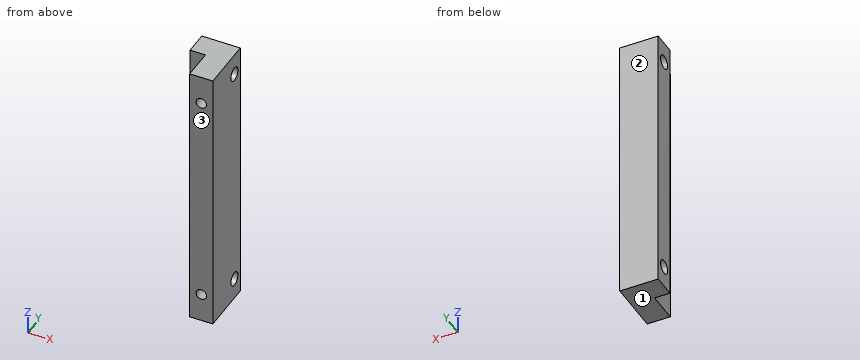
from build123d import *

# Parameters (mm, degrees)
AUFSATZ_LINEAR_AUSTRAGEN1_DEPTH = 89
M8_GEWINDEBOHRUNG1_D            = 6.8
M8_GEWINDEBOHRUNG1_DEPTH        = 18.25
M8_GEWINDEBOHRUNG1_TIP          = 2.042926105
F_9_0_9_DURCHMESSER_BOHRUNG1_D  = 9


with BuildPart() as part:
    # Skizze1 → Aufsatz-Linear austragen1 (new, symmetric)
    with BuildSketch(Plane.XY):
        Polygon((0, 0), (15, 0), (15, 35), (-10, 35), (-10, 20), (0, 20), align=None)
    extrude(amount=AUFSATZ_LINEAR_AUSTRAGEN1_DEPTH, both=True)

    # M8 Gewindebohrung1
    with Locations(Plane(origin=(0, 0, 0), x_dir=(-1, 0, 0), z_dir=(0, -1, 0))):
        with Locations((-7.5, -70), (-7.5, 70)):
            Hole(M8_GEWINDEBOHRUNG1_D / 2, depth=M8_GEWINDEBOHRUNG1_DEPTH)
            with Locations((0, 0, -(M8_GEWINDEBOHRUNG1_DEPTH + M8_GEWINDEBOHRUNG1_TIP / 2))):  # 118° drill point
                Cone(0, M8_GEWINDEBOHRUNG1_D / 2, M8_GEWINDEBOHRUNG1_TIP, mode=Mode.SUBTRACT)

    # Ø9.0 (9) Durchmesser Bohrung1 (through all)
    with Locations(Plane(origin=(15, 0, 0), x_dir=(0, 0, -1), z_dir=(1, 0, 0))):
        with Locations((-75, 27.5), (75, 27.5)):
            Hole(F_9_0_9_DURCHMESSER_BOHRUNG1_D / 2)


solid = part.part
Here's how the part is built. I have some questions about the finished solid (model axes, mm). Face numbers are marked on the shaded views. Round coordinates to 2 decimals unless told otherwise and drop trailing zeros. Order: outer loops, then holes, each group sorted by start corner. A loop starts at its lowest first (then second) coordinate and runs counter-clockwise, first axis right, second up. Notation, with made-up numbers: M -30,59.5 L 15,59.5 A19 cw 15,95.5 Z; hole C 48,80.25 d6. An arc over 180 degrees is marked long. Return JSON: item names as keys, results as strings. Group by question number.
1. If we section it at C-C on y = 14: List the corners of the cut face in (x, z) for me, then the cut area to 3 significant figures.
2. Please list where these lines run through material, in increasing order: probe 1 along Z at (x, y) = (7.5, 14.25); probe 2 along X at (y, z) = (5, -70); probe 3 along Y at (x, z) = (2.25, 75).
3. If we section it at B-B on z = -75: List the corners of the cut face in (x, y) for me, then the cut area to 3 significant figures.
4. If we section it at D-D on x = -5: List the corners of the cut face in (y, z) for me, then the cut area to 3 significant figures.
5. If we mould it in two halves opening along Y, with no side actions, what happens to the marked faces 1, 2 and 3? For each: pulls with the +Y half, pulls with the -Y half, needs draft (parallel to the pull), parting line crosses it, or undercut.
6. I'm going to push flat-ended pins straight in: pin 1 Ø3 at (x, z) = (-3.5, -28.5) entering from -Y; pin 2 Ø4 at (x, z) = (7.5, 70) entering from -Y; pin 3 Ø6 at (y, z) = (14, -4.5) entering from -X; pin 4 Ø7 at (y, z) = (27.5, 75) entering from -X. Where does each tip first touch, or does it pass through?
7. If we section it at A-A on y = 27.5: List the corners of the cut face in (x, z) for me, then the cut area to 3 significant figures.
Reply:
{
 "1": {"outline": "M 0,-89 L 15,-89 L 15,89 L 0,89 Z; hole C 7.5,-70 d6.8; hole C 7.5,70 d6.8", "area": "2,600 mm^2"},
 "2": {"probe 1": "-89 to -73.4, -66.6 to 66.6, 73.4 to 89", "probe 2": "0 to 4.1, 10.9 to 15", "probe 3": "0 to 23, 32 to 35"},
 "3": {"outline": "M -10,20 L 0,20 L 0,0 L 15,0 L 15,23 L -10,23 Z; M -10,32 L 15,32 L 15,35 L -10,35 Z", "area": "450 mm^2"},
 "4": {"outline": "M 20,-89 L 35,-89 L 35,89 L 20,89 Z; hole C 27.5,-75 d9; hole C 27.5,75 d9", "area": "2,540 mm^2"},
 "5": {"face 1": "needs draft", "face 2": "pulls with the +Y half", "face 3": "pulls with the -Y half"},
 "6": {"pin 1": "y = 20", "pin 2": "y = 19.09", "pin 3": "x = 0", "pin 4": "through"},
 "7": {"outline": "M -10,-89 L 15,-89 L 15,-79.5 L -10,-79.5 Z; M -10,-70.5 L 15,-70.5 L 15,70.5 L -10,70.5 Z; M -10,79.5 L 15,79.5 L 15,89 L -10,89 Z", "area": "4,000 mm^2"}
}
